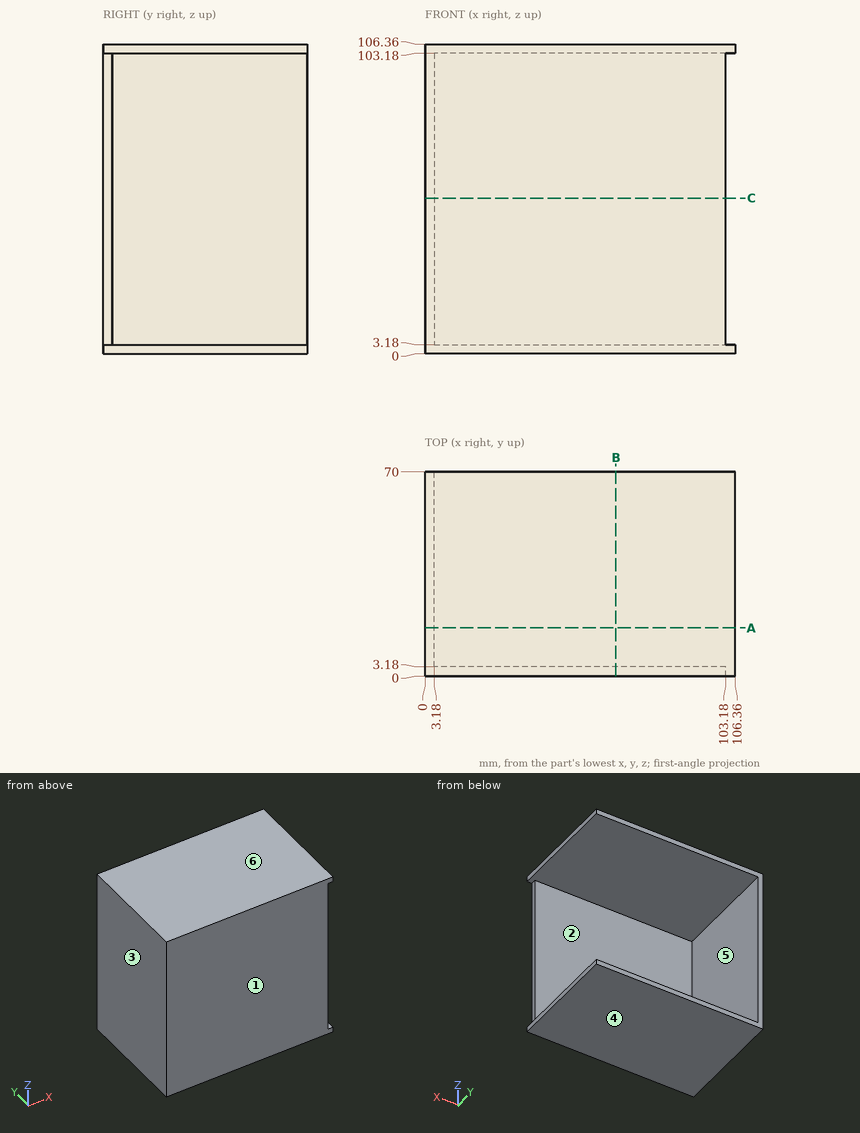
Verification items for this drawing (mm, ordinates from the low corner). A direction names the side the tool comes from. Coordinates: 2 decimals unless noted, no trailing zeros. Write each loop counter-clockwise with the first axis right and the second up, starting at its lowest first coordinate (ties: lowest second). Pieces come first, ordered by that corner, then holes. Notation, with made-up numbers: (80.25, -15.75) -> (138.25, -15.75) arc R13 cw to (138.25, -3.75) -> close; hole circle Ø11 at (69.25, 56). An arc over 180 degrees is marked (long way). Use CSV: the item, a comma, the result in double quotes. Start each with the question number.
Item 1: Mould release check, pull along Z, two halves, no side actions. Record for the marked faces 3, 4, 5 and 6: released by +Z, released by -Z, zero draft, split by the parting line, or undercut.
Item 2: Set-up check for the marked faces 1 and 2: record each of +Z, -Z, +X, -X, +Y, -Y from which the full face is reachable in a straight line by a thin tool's end or side.
Item 3: Thickness scan on line 1 (Z direction, x = 95, y = 23.5); line 2 (X direction, y = 5.5, z = 98). Record the ranges inside material, lowest first.
Item 4: Cross-section at A-A, the plane y = 16.5. Record the cut outline in (x, z).
Item 5: Cross-section at C-C, the plane z = 53.5. Record the cut outline in (x, y).
Item 6: Cross-section at B-B, the plane x = 65.5. Record the cut outline in (y, z), plus the area to 3 significant figures.
Item 7: Depth check by flat-ended pin: pin 1 Ø2 at (y, z) = (7.5, 44) entering from +X; pin 2 Ø1 at (y, z) = (2, 35.5) entering from +X. Enter the tip coordinate at first touch or a pass-through.
Answers:
1,face 3,"zero draft"
1,face 4,"released by -Z"
1,face 5,"undercut"
1,face 6,"released by +Z"
2,face 1,"+Z, -Z, +X, -X, -Y"
2,face 2,"+X, +Y"
3,line 1,"0 to 3.18, 103.18 to 106.36"
3,line 2,"0 to 3.18"
4,outline,"(0, 0) -> (106.36, 0) -> (106.36, 3.18) -> (3.18, 3.18) -> (3.18, 103.18) -> (106.36, 103.18) -> (106.36, 106.36) -> (0, 106.36) -> close"
5,outline,"(0, 0) -> (103.18, 0) -> (103.18, 3.18) -> (3.18, 3.18) -> (3.18, 70) -> (0, 70) -> close"
6,outline,"(0, 0) -> (70, 0) -> (70, 3.18) -> (3.18, 3.18) -> (3.18, 103.18) -> (70, 103.18) -> (70, 106.36) -> (0, 106.36) -> close"
6,area,"763 mm^2"
7,pin 1,"x = 3.18"
7,pin 2,"x = 103.18"
